The model under review builds one solid part; all positions refer to its coordinate system, in mm. A direction names the side the tool comes from. Coordinates: 2 decimals unless noted, no trailing zeros. Order: outer loops, then holes, each group sorted by start corner. A loop starts at its lowest first (then second) coordinate and runs counter-clockwise, first axis right, second up. Notation, with made-up numbers: M 82,-22.75 L 104,-22.75 A26 cw 104,-8.75 Z; hole C 74,39.5 d11. An arc over 180 degrees is marked long. Write each question's results on one line, items separated by ' | '.
from build123d import *

# Parameters (mm, degrees)
F1_DEPTH = 2
F2_R     = 3.55
F3_DEPTH = 25
F5_DEPTH = 4


with BuildPart() as f1:
    # F0 (on Top) → F1 (new body)
    with BuildSketch(Plane.XY):
        with BuildLine():
            ThreePointArc((9.165151, -5.9), (10.457298, -3.074886), (10.9, 0))
            ThreePointArc((10.9, 0), (10.457298, 3.074886), (9.165151, 5.9))
            Line((9.165151, 5.9), (-9.165151, 5.9))
            ThreePointArc((-9.165151, 5.9), (-10.9, 0), (-9.165151, -5.9))
            Line((-9.165151, -5.9), (9.165151, -5.9))
        make_face()
    extrude(amount=F1_DEPTH)

    # F2 (on face) → F3 (cut)
    with BuildSketch(Plane.XY.offset(2)):
        Circle(F2_R)
    extrude(amount=-F3_DEPTH, mode=Mode.SUBTRACT)

    # F4 (on face) → F5 (join)
    with BuildSketch(Plane.XY.offset(2)):
        with BuildLine():
            Line((-10.099505, 4.1), (10.099505, 4.1))
            ThreePointArc((10.099505, 4.1), (9.674283, 5.021778), (9.165151, 5.9))
            Line((9.165151, 5.9), (-9.165151, 5.9))
            ThreePointArc((-9.165151, 5.9), (-9.674283, 5.021778), (-10.099505, 4.1))
        make_face()
        with BuildLine():
            ThreePointArc((9.165151, -5.9), (9.674283, -5.021778), (10.099505, -4.1))
            Line((10.099505, -4.1), (-10.099505, -4.1))
            ThreePointArc((-10.099505, -4.1), (-9.674283, -5.021778), (-9.165151, -5.9))
            Line((-9.165151, -5.9), (9.165151, -5.9))
        make_face()
    extrude(amount=F5_DEPTH)


solid = f1.part
1) Take a section at B-B on z = 3.1. State the section outline as (x, y) points, plus the area to 3 significant figures.
Solutions:
outline: M -10.1,-4.1 A10.9 ccw -9.17,-5.9 L 9.17,-5.9 A10.9 ccw 10.1,-4.1 Z; M -10.1,4.1 L 10.1,4.1 A10.9 ccw 9.17,5.9 L -9.17,5.9 A10.9 ccw Z | area: 69.6 mm2
2) For faces 4 (the flat face through (0, -5.9, 3)), 5 (the flat face through (-3, 3, 2)), list the 3-axis set-ups (+Z, -Z, +X, -X, +Y, -Y) from which the entire face can be reached by the end or side of a thin tool; tool diameter is ignored.
Solutions:
face 4: +Z, -Z, +X, -X, -Y | face 5: +Z, +X, -X
3) The part is to be moulded in two halves that separate along Y. For faces 1 (the flat face through (0, -4.1, 4)), 2 (the flat face through (0, 5.9, 3)), 3 (the cylindrical face through (9.67, -5.03, 3.97)), say which applies: pulls with the +Y half, pulls with the -Y half, needs draft (parallel to the pull), parting line crosses it, or undercut.
Solutions:
face 1: undercut | face 2: pulls with the +Y half | face 3: pulls with the -Y half
4) To check wall thickness, follow line 1 along Y through (x, z) = (0, 0.8); line 2 along Z through (x, y) = (9.25, -1); line 3 along Y through (x, z) = (9.5, 2.4). State the ranges of each line that lie inside material, in increasing order.
Solutions:
line 1: -5.9 to -3.55, 3.55 to 5.9 | line 2: 0 to 2 | line 3: -5.34 to -4.1, 4.1 to 5.34
5) Take a section at D-D on x = 7.75. State the section outline as (y, z) points, plus the area to 3 significant figures.
Solutions:
outline: M -5.9,0 L 5.9,0 L 5.9,6 L 4.1,6 L 4.1,2 L -4.1,2 L -4.1,6 L -5.9,6 Z | area: 38.0 mm2
6) Take a section at A-A on x = 0. State the section outline as (y, z) points.
Solutions:
outline: M -5.9,0 L -3.55,0 L -3.55,2 L -4.1,2 L -4.1,6 L -5.9,6 Z; M 3.55,0 L 5.9,0 L 5.9,6 L 4.1,6 L 4.1,2 L 3.55,2 Z
7) Take a section at C-C on y = 2.75. State the section outline as (x, z) points (3 decimals), plus the area to 3 significant figures.
Solutions:
outline: M -10.547,0 L -2.245,0 L -2.245,2 L -10.547,2 Z; M 2.245,0 L 10.547,0 L 10.547,2 L 2.245,2 Z | area: 33.2 mm2
